from build123d import *

# Parameters (mm, degrees)
BOSS_EXTRU_2_DEPTH = 316.8


with BuildPart() as part:
    # Esquisse1_3 → Boss.-Extru.2 (new body)
    with BuildSketch(Plane(origin=(0, 0, 0), x_dir=(1, 0, 0), z_dir=(0, 1, 0))):
        Polygon((17.5, 2.5), (13.964466094, 2.5), (16.464466094, 0), (20, 0), (20, 3.535533906), (17.5, 6.035533906), align=None)
        Polygon((16.464466094, 0), (13.964466094, 2.5), (13.964466094, 0), align=None)
        Polygon((20, 6.035533906), (17.5, 6.035533906), (20, 3.535533906), align=None)
        Polygon((13.964466094, 20), (13.964466094, 17.5), (16.464466094, 20), align=None)
        Polygon((20, 16.464466094), (17.5, 13.964466094), (20, 13.964466094), align=None)
        Polygon((16.464466094, 20), (13.964466094, 17.5), (17.5, 17.5), (17.5, 13.964466094), (20, 16.464466094), (20, 20), align=None)
        Polygon((13.535533906, 10), (10, 6.464466094), (13.964466094, 2.5), (17.5, 2.5), (17.5, 6.035533906), align=None)
        Polygon((10, 13.535533906), (6.464466094, 10), (10, 6.464466094), (13.535533906, 10), align=None)
        Polygon((13.964466094, 17.5), (10, 13.535533906), (13.535533906, 10), (17.5, 13.964466094), (17.5, 17.5), align=None)
        Polygon((6.464466094, 10), (2.5, 6.035533906), (2.5, 2.5), (6.035533906, 2.5), (10, 6.464466094), align=None)
        Polygon((2.5, 6.035533906), (0, 3.535533906), (3.535533906, 0), (6.035533906, 2.5), (2.5, 2.5), align=None)
        Polygon((3.535533906, 0), (0, 3.535533906), (0, 0), align=None)
        Polygon((0, 0), (0, 3.535533906), (-3.535533906, 0), align=None)
        Polygon((0, 3.535533906), (-2.5, 6.035533906), (-2.5, 2.5), (-6.035533906, 2.5), (-3.535533906, 0), align=None)
        Polygon((0, 6.035533906), (-2.5, 6.035533906), (0, 3.535533906), align=None)
        Polygon((0, 6.035533906), (0, 3.535533906), (2.5, 6.035533906), align=None)
        Polygon((-3.535533906, 0), (-6.035533906, 2.5), (-6.035533906, 0), align=None)
        Polygon((6.035533906, 2.5), (3.535533906, 0), (6.035533906, 0), align=None)
        Polygon((-2.5, 2.5), (-2.5, 6.035533906), (-6.464466094, 10), (-10, 6.464466094), (-6.035533906, 2.5), align=None)
        Polygon((0, 16.464466094), (-2.5, 13.964466094), (0, 13.964466094), align=None)
        Polygon((2.5, 13.964466094), (0, 16.464466094), (0, 13.964466094), align=None)
        Polygon((3.535533906, 20), (0, 16.464466094), (2.5, 13.964466094), (2.5, 17.5), (6.035533906, 17.5), align=None)
        Polygon((6.035533906, 20), (3.535533906, 20), (6.035533906, 17.5), align=None)
        Polygon((0, 20), (0, 16.464466094), (3.535533906, 20), align=None)
        Polygon((-6.035533906, 17.5), (-2.5, 17.5), (-2.5, 13.964466094), (0, 16.464466094), (-3.535533906, 20), align=None)
        Polygon((0, 20), (-3.535533906, 20), (0, 16.464466094), align=None)
        Polygon((-6.035533906, 20), (-6.035533906, 17.5), (-3.535533906, 20), align=None)
        Polygon((-2.5, 13.964466094), (-2.5, 17.5), (-6.035533906, 17.5), (-10, 13.535533906), (-6.464466094, 10), align=None)
        Polygon((-6.464466094, 10), (-10, 13.535533906), (-13.535533906, 10), (-10, 6.464466094), align=None)
        Polygon((-16.464466094, 20), (-13.964466094, 17.5), (-13.964466094, 20), align=None)
        Polygon((-17.5, 17.5), (-13.964466094, 17.5), (-16.464466094, 20), (-20, 20), (-20, 16.464466094), (-17.5, 13.964466094), align=None)
        Polygon((-20, 13.964466094), (-17.5, 13.964466094), (-20, 16.464466094), align=None)
        Polygon((-10, 13.535533906), (-13.964466094, 17.5), (-17.5, 17.5), (-17.5, 13.964466094), (-13.535533906, 10), align=None)
        Polygon((-20, 3.535533906), (-17.5, 6.035533906), (-20, 6.035533906), align=None)
        Polygon((-13.964466094, 0), (-13.964466094, 2.5), (-16.464466094, 0), align=None)
        Polygon((-17.5, 2.5), (-17.5, 6.035533906), (-20, 3.535533906), (-20, 0), (-16.464466094, 0), (-13.964466094, 2.5), align=None)
        Polygon((-10, 6.464466094), (-13.535533906, 10), (-17.5, 6.035533906), (-17.5, 2.5), (-13.964466094, 2.5), align=None)
        Polygon((2.5, 17.5), (2.5, 13.964466094), (6.464466094, 10), (10, 13.535533906), (6.035533906, 17.5), align=None)
    extrude(amount=BOSS_EXTRU_2_DEPTH)


solid = part.part
Here's how the part is built. I have some questions about the finished solid (model axes, mm). Give positions to 0.01 mm unless a question says otherwise; leave off trailing zeros. Use one line per item in the form item = value. Start each with the question number.
1. Will this pin go through, and if not, where does the flat tip stop? pin 1 Ø2 at (y, z) = (244.5, -10.5) entering from +X.
2. If I drill on L1, parallel to X at y = 118.5, z = -19; L2, parallel to Z at x = -1.5, y = 187.5; L3, parallel to X at y = 91, z = -5.75, over which ranges is the centre line in solid material (lowest first)?
3. Thinking about a two-plate mould opening in X: for faces 1 (the face through (0, 156, -6.036)), 2 (the face through (0, 156, -13.964)), 3 (the face through (20, 156, -17)), 4 (the face through (-17, 156, 0)), which applies, +X half, -X half, draft (parallel to the pull), parting line (faces both ways), or undercut?
Entries:
q1.pin_1 = 15.04
q2.L1 = -20 to -13.96, -6.04 to 6.04, 13.96 to 20
q2.L2 = -20 to -13.96, -6.04 to 0
q2.L3 = -20 to -10.71, -9.29 to 9.29, 10.71 to 20
q3.face_1 = undercut
q3.face_2 = undercut
q3.face_3 = +X half
q3.face_4 = draft
